Source: CAD feature listing. Evaluate the final solid. Frame: model axes, mm. A direction names the side the tool comes from. Coordinates: 2 decimals unless noted, no trailing zeros. Write each loop counter-clockwise with the first axis right and the second up, starting at its lowest first coordinate (ties: lowest second). Pieces come first, ordered by that corner, then holes. Notation, with made-up numbers: (13.5, 65.5) - (37.5, 65.5) arc R9 cw to (37.5, 79.5) - close; hole circle Ø8 at (-33, 63). An arc over 180 degrees is marked (long way). One line per question, with ' | ' between items.
Autodesk Inventor part; units mm, degrees
ref_plane "YZ Plane" through (0, 0, 0) normal (1, 0, 0) x (0, 1, 0)
ref_plane "XZ Plane" through (0, 0, 0) normal (0, 1, 0) x (-1, 0, 0)
ref_plane "XY Plane" through (0, 0, 0) normal (0, 0, 1) x (1, 0, 0)
sketch "スケッチ1" plane through (0, 0, 0) normal (0, 1, 0) x (-1, 0, 0)
  circle A0 centre (0, 0) radius 10
  dimension "d0" = 20
extrude "押し出し1" add sketch "スケッチ1" along normal blind 2
sketch "スケッチ2" plane through (0, 2, 0) normal (0, 1, 0) x (1, 0, 0)
  circle A0 centre (0, 0) radius 7 construction
  circle A1 centre (-7, 0) radius 1
  circle A2 centre (-4.9497, -4.9497) radius 1
  circle A3 centre (0, -7) radius 1
  circle A4 centre (4.9497, -4.9497) radius 1
  circle A5 centre (7, 0) radius 1
  circle A6 centre (4.9497, 4.9497) radius 1
  circle A7 centre (-4.9497, 4.9497) radius 1
  circle A8 centre (0, 7) radius 1
  dimension "d3" = 14
  dimension "d4" = 2
  dimension "d5" = 2
  dimension "d6" = 2
  dimension "d7" = 2
  dimension "d8" = 2
  dimension "d9" = 2
  dimension "d10" = 2
  dimension "d11" = 2
extrude "押し出し2" cut sketch "スケッチ2" against normal blind 2
sketch "スケッチ3" plane through (0, 2, 0) normal (0, 1, 0) x (1, 0, 0)
  circle A0 centre (0, 0) radius 5
  dimension "d14" = 10
extrude "押し出し3" add sketch "スケッチ3" along normal blind 1
sketch "スケッチ4" plane through (0, 3, 0) normal (0, 1, 0) x (1, 0, 0)
  circle A0 centre (0, 0) radius 1.6
  dimension "d17" = 3.2
extrude "押し出し4" cut sketch "スケッチ4" against normal blind 1
sketch "スケッチ5" plane through (0, 0, 0) normal (0, -1, 0) x (1, 0, 0)
  circle A0 centre (0, 0) radius 5
  dimension "d20" = 10
extrude "押し出し5" add sketch "スケッチ5" along normal blind 1
sketch "スケッチ6" plane through (0, -1, 0) normal (0, -1, 0) x (1, 0, 0)
  circle A0 centre (0, 0) radius 3
  dimension "d23" = 6
extrude "押し出し6" cut sketch "スケッチ6" against normal blind 3
properties part number "ServoHorn"
Item 1: Mould query, pull axis X, two halves, no side actions, for faces 4 (the face through (3.3, -1, 0.1)), 5 (the face through (-1.08, 2.49, -4.88)), 6 (the face through (-7.8, 1, 0.6)). Classes: pulls with the +X half, pulls with the -X half, needs draft (parallel to the pull), parting line crosses it, or undercut.
Check sheet entries:
face 4: needs draft | face 5: parting line crosses it | face 6: undercut
Item 2: Cut plane A-A on x = 0. Return loops of the section in (y, z), and give its area (3 significant figures).
Check sheet entries:
outline: (-1, -5) - (0, -5) - (0, -6) - (2, -6) - (2, -5) - (3, -5) - (3, -1.6) - (2, -1.6) - (2, -3) - (-1, -3) - close; (-1, 3) - (2, 3) - (2, 1.6) - (3, 1.6) - (3, 5) - (2, 5) - (2, 6) - (0, 6) - (0, 5) - (-1, 5) - close; (0, -10) - (2, -10) - (2, -8) - (0, -8) - close; (0, 8) - (2, 8) - (2, 10) - (0, 10) - close | area: 30.8 mm²
Item 3: Cut plane B-B on z = 7. Return loops of the section in (x, y), and give its area (3 significant figures).
Check sheet entries:
outline: (-7.14, 0) - (-1, 0) - (-1, 2) - (-7.14, 2) - close; (1, 0) - (7.14, 0) - (7.14, 2) - (1, 2) - close | area: 24.6 mm²
Item 4: Pin query (flat end, axial travel): pin 1 Ø4 at (x, z) = (0, 0) entering from +Y; pin 2 Ø1.8 at (x, z) = (7, 0) entering from -Y; pin 3 Ø2.5 at (x, z) = (-7, 0) entering from +Y; pin 4 Ø1.8 at (x, z) = (-0.5, 1) entering from -Y. Return the tip coordinate at first contact, or that it passes through.
Check sheet entries:
pin 1: y = 3 | pin 2: through | pin 3: y = 2 | pin 4: y = 2
Item 5: Cut plane C-C on z = 0. Return loops of the section in (x, y).
Check sheet entries:
outline: (-10, 0) - (-8, 0) - (-8, 2) - (-10, 2) - close; (-6, 0) - (-5, 0) - (-5, -1) - (-3, -1) - (-3, 2) - (-1.6, 2) - (-1.6, 3) - (-5, 3) - (-5, 2) - (-6, 2) - close; (1.6, 2) - (3, 2) - (3, -1) - (5, -1) - (5, 0) - (6, 0) - (6, 2) - (5, 2) - (5, 3) - (1.6, 3) - close; (8, 0) - (10, 0) - (10, 2) - (8, 2) - close
Item 6: Cut plane D-D on y = -0.35. Return loops of the section in (x, z), and give its area (3 significant figures).
Check sheet entries:
outline: circle Ø10 at (0, 0); hole circle Ø6 at (0, 0) | area: 50.3 mm²
Item 7: Ray query, line 1 along Z through (x, y) = (0, 0.9); line 2 along Z through (x, y) = (0, 2.8); line 3 along Z through (x, y) = (0.75, 0.6). Return the intervals inside material, ascending. Write a range as [from, to].
Check sheet entries:
line 1: [-10, -8], [-6, -3], [3, 6], [8, 10] | line 2: [-5, -1.6], [1.6, 5] | line 3: [-9.97, -7.66], [-6.34, -2.9], [2.9, 6.34], [7.66, 9.97]
Item 8: Access query for faces 1 (the face through (-2, 0, 5)), 2 (the face through (0, 1, -8)), 3 (the face through (-2, 2, 5)). Directions: +Z, -Z, +X, -X, +Y, -Y. A direction counts if a zero-diameter tool reaches every point of the face in a straight line with its end or side. Return the directions, or none.
Check sheet entries:
face 1: -Y | face 2: +Y, -Y | face 3: +Y
